```python
from build123d import *

# Parameters (mm, degrees)
ESQUISSE1_R        = 11.5
ESQUISSE1_R_2      = 1.6
BOSS_EXTRU_1_DEPTH = 4.8


with BuildPart() as part:
    # Esquisse1 → Boss.-Extru.1 (new body)
    with BuildSketch(Plane(origin=(0, 0, 0), x_dir=(-1, 0, 0), z_dir=(0, 0, -1))):
        with BuildLine():
            Line((0, 9.500081158), (0, 49.000418249))
            ThreePointArc((0, 49.000418249), (-1.464478579, 52.535982296), (-5.000042626, 54.000460875))
            Line((-5.000042626, 54.000460875), (-68.000581364, 54.000460875))
            ThreePointArc((-68.000581364, 54.000460875), (-71.53614516, 52.535982401), (-73.000623635, 49.000418605))
            Line((-73.000623635, 49.000418605), (-73.000623635, 9.500081158))
            ThreePointArc((-73.000623635, 9.500081158), (-72.854175775, 9.146524747), (-72.500619364, 9.000076887))
            Line((-72.500619364, 9.000076887), (-47.250403654, 9.000076887))
            Line((-47.250403654, 9.000076887), (-47.250403654, 1.000007743))
            ThreePointArc((-47.250403654, 1.000007743), (-46.95750587, 0.292889941), (-46.250388068, -7.843e-06))
            Line((-46.250388068, -7.843e-06), (-26.75023547, -7.843e-06))
            ThreePointArc((-26.75023547, -7.843e-06), (-26.043121781, 0.292888237), (-25.750225701, 1.000001925))
            Line((-25.750225701, 1.000001925), (-25.750225701, 9.000076887))
            Line((-25.750225701, 9.000076887), (-0.500004271, 9.000076887))
            ThreePointArc((-0.500004271, 9.000076887), (-0.14644786, 9.146524747), (0, 9.500081158))
        make_face()
        with Locations((-36.5004012, 30.150219609)):
            Circle(ESQUISSE1_R, mode=Mode.SUBTRACT)
        with Locations((-52.0004012, 14.650219609)):
            Circle(ESQUISSE1_R_2, mode=Mode.SUBTRACT)
        with Locations((-52.000444233, 45.650219609)):
            Circle(ESQUISSE1_R_2, mode=Mode.SUBTRACT)
        with Locations((-21.0004012, 14.650219609)):
            Circle(ESQUISSE1_R_2, mode=Mode.SUBTRACT)
        with Locations((-21.0004012, 45.650219609)):
            Circle(ESQUISSE1_R_2, mode=Mode.SUBTRACT)
        Polygon((-6.200052966, 47.036041823), (-5.614406963, 46.45039682), (-5.400046132, 45.650389986), (-5.614406963, 44.850383151), (-6.200052966, 44.264738148), (-7.000059801, 44.050376317), (-7.800066635, 44.264738148), (-8.385711638, 44.850383151), (-8.600073469, 45.650389986), (-8.385711638, 46.45039682), (-7.800066635, 47.036041823), (-7.000059801, 47.250403654), align=None, mode=Mode.SUBTRACT)
        Polygon((-4.750040579, 35.000299003), (-4.716546293, 35.125300071), (-4.625039511, 35.216810853), (-4.500038443, 35.250301139), (-4.375037375, 35.216810853), (-4.283530594, 35.125300071), (-4.250036308, 35.000299003), (-4.283530594, 34.875297935), (-4.375037375, 34.783787154), (-4.500038443, 34.750296868), (-4.500038443, 25.250215709), (-4.375037375, 25.216725423), (-4.283530594, 25.125214642), (-4.250036308, 25.000213574), (-4.283530594, 24.875212506), (-4.375037375, 24.783701724), (-4.500038443, 24.750211438), (-4.625039511, 24.783701724), (-4.716546293, 24.875212506), (-4.750040579, 25.000213574), (-9.250079022, 25.000213574), (-9.283572308, 24.875212506), (-9.37508009, 24.783701724), (-9.500081158, 24.750211438), (-9.625082226, 24.783701724), (-9.716589008, 24.875212506), (-9.750083294, 25.000213574), (-9.716589008, 25.125214642), (-9.625082226, 25.216725423), (-9.500081158, 25.250215709), (-9.500081158, 34.750296868), (-9.625082226, 34.783787154), (-9.716589008, 34.875297935), (-9.750083294, 35.000299003), (-9.716589008, 35.125300071), (-9.625082226, 35.216810853), (-9.500081158, 35.250301139), (-9.37508009, 35.216810853), (-9.283572308, 35.125300071), (-9.250079022, 35.000299003), align=None, mode=Mode.SUBTRACT)
        Polygon((-5.614406963, 15.450131989), (-5.400046132, 14.650125154), (-5.614406963, 13.85011832), (-6.200052966, 13.264473317), (-7.000059801, 13.050111485), (-7.800066635, 13.264473317), (-8.385711638, 13.85011832), (-8.600073469, 14.650125154), (-8.385711638, 15.450131989), (-7.800066635, 16.035776992), (-7.000059801, 16.250138823), (-6.200052966, 16.035776992), align=None, mode=Mode.SUBTRACT)
        Polygon((-30.100257143, 1.874182011), (-30.750262696, 1.700013523), (-31.400268249, 1.874182011), (-31.876102314, 2.350020076), (-32.050273802, 3.000025629), (-31.876102314, 3.650030182), (-31.400268249, 4.125868247), (-30.750262696, 4.300036735), (-30.100257143, 4.125868247), (-29.624423078, 3.650030182), (-29.45025159, 3.000025629), (-29.624423078, 2.350020076), align=None, mode=Mode.SUBTRACT)
        Polygon((-39.600338301, 1.874182011), (-40.250343854, 1.700013523), (-40.900349407, 1.874182011), (-41.376193472, 2.350020076), (-41.55035496, 3.000025629), (-41.376193472, 3.650030182), (-40.900349407, 4.125868247), (-40.250343854, 4.300036735), (-39.600338301, 4.125868247), (-39.124504236, 3.650030182), (-38.950332748, 3.000025629), (-39.124504236, 2.350020076), align=None, mode=Mode.SUBTRACT)
        Polygon((-64.400550166, 14.650125154), (-64.614911997, 13.85011832), (-65.200557, 13.264473317), (-66.000563835, 13.050111485), (-66.800570669, 13.264473317), (-67.386215672, 13.85011832), (-67.600577503, 14.650125154), (-67.386215672, 15.450131989), (-66.800570669, 16.035776992), (-66.000563835, 16.250138823), (-65.200557, 16.035776992), (-64.614911997, 15.450131989), align=None, mode=Mode.SUBTRACT)
        Polygon((-63.625543545, 24.783701724), (-63.717054327, 24.875212506), (-63.750544613, 25.000213574), (-68.250583056, 25.000213574), (-68.284073342, 24.875212506), (-68.375584124, 24.783701724), (-68.500585192, 24.750211438), (-68.62558626, 24.783701724), (-68.717097042, 24.875212506), (-68.750587328, 25.000213574), (-68.717097042, 25.125214642), (-68.62558626, 25.216725423), (-68.500585192, 25.250215709), (-68.500585192, 34.750296868), (-68.62558626, 34.783787154), (-68.717097042, 34.875297935), (-68.750587328, 35.000299003), (-68.717097042, 35.125300071), (-68.62558626, 35.216810853), (-68.500585192, 35.250301139), (-68.375584124, 35.216810853), (-68.284073342, 35.125300071), (-68.250583056, 35.000299003), (-63.750544613, 35.000299003), (-63.717054327, 35.125300071), (-63.625543545, 35.216810853), (-63.500542477, 35.250301139), (-63.375541409, 35.216810853), (-63.284040628, 35.125300071), (-63.250540342, 35.000299003), (-63.284040628, 34.875297935), (-63.375541409, 34.783787154), (-63.500542477, 34.750296868), (-63.500542477, 25.250215709), (-63.375541409, 25.216725423), (-63.284040628, 25.125214642), (-63.250540342, 25.000213574), (-63.284040628, 24.875212506), (-63.375541409, 24.783701724), (-63.500542477, 24.750211438), align=None, mode=Mode.SUBTRACT)
        Polygon((-66.800570669, 47.036041823), (-66.000563835, 47.250403654), (-65.200557, 47.036041823), (-64.614911997, 46.45039682), (-64.400550166, 45.650389986), (-64.614911997, 44.850383151), (-65.200557, 44.264738148), (-66.000563835, 44.050376317), (-66.800570669, 44.264738148), (-67.386215672, 44.850383151), (-67.600577503, 45.650389986), (-67.386215672, 46.45039682), align=None, mode=Mode.SUBTRACT)
    extrude(amount=-BOSS_EXTRU_1_DEPTH)


solid = part.part
```
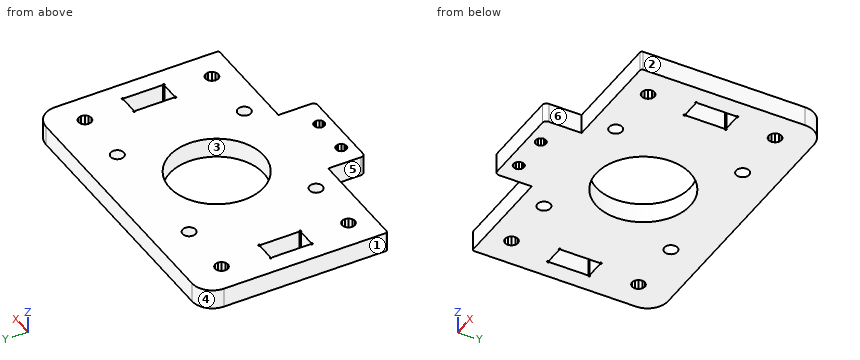
Source: CAD feature listing. Evaluate the final solid. Frame: model axes, mm. Face numbers are marked on the shaded views. A direction names the side the tool comes from. Give positions to 0.01 mm unless a question says otherwise; leave off trailing zeros. Write each loop counter-clockwise with the first axis right and the second up, starting at its lowest first coordinate (ties: lowest second). Pieces come first, ordered by that corner, then holes.
1. Section query D-D (x = 52.5). Return the cut outline in (y, z).
2. Section query A-A (x = 37). Return the cut outline in (y, z).
3. Section query C-C (y = 34). Return the cut outline in (x, z).
4. Section query B-B (y = 20). Return the cut outline in (x, z), then the cut area to 3 significant figures.
5. Material intervals for line 1 along X through (y, z) = (15.5, 3.45); line 2 along Y through (x, z) = (37, 0.4); line 3 along X through (y, z) = (33, 0.45), sorted ascending.
6. Pull-direction query (X, two-part tool) for the marked faces 1, 2 and 3; classes: +X half, -X half, draft (parallel to the pull), parting line (faces both ways), or undercut.
7. First-contact query: pin 1 (1.5 mm diameter, centred on x = 62.5, z = 2, fed in from -Y). Flat tip, straight axial feed; report the tip coordinate or a pass-through.
8. Access query for the marked faces 4, 5 and 6. Directions: +Z, -Z, +X, -X, +Y, -Y. A direction counts if a zero-diameter tool reaches every point of the face in a straight line with its end or side. Return the directions, or none.
Output values:
1. outline: (9, 0) - (13.13, 0) - (13.13, 4.8) - (9, 4.8) - close; (16.17, 0) - (44.13, 0) - (44.13, 4.8) - (16.17, 4.8) - close; (47.17, 0) - (54, 0) - (54, 4.8) - (47.17, 4.8) - close
2. outline: (0, 0) - (18.66, 0) - (18.66, 4.8) - (0, 4.8) - close; (41.64, 0) - (54, 0) - (54, 4.8) - (41.64, 4.8) - close
3. outline: (0, 0) - (4.5, 0) - (4.5, 4.8) - (0, 4.8) - close; (9.5, 0) - (25.66, 0) - (25.66, 4.8) - (9.5, 4.8) - close; (47.34, 0) - (63.5, 0) - (63.5, 4.8) - (47.34, 4.8) - close; (68.5, 0) - (73, 0) - (73, 4.8) - (68.5, 4.8) - close
4. outline: (0, 0) - (31.09, 0) - (31.09, 4.8) - (0, 4.8) - close; (41.91, 0) - (73, 0) - (73, 4.8) - (41.91, 4.8) - close
4. area: 299 mm2
5. line 1: x = 0 to 5.66, 8.34 to 19.64, 22.36 to 50.64, 53.36 to 64.66, 67.34 to 73
5. line 2: y = 0 to 18.66, 41.64 to 54
5. line 3: x = 0 to 4.5, 9.5 to 25.36, 47.64 to 63.5, 68.5 to 73
6. face 1: -X half
6. face 2: +X half
6. face 3: undercut
7. pin 1: stops at y = 9
8. face 4: +Z, -Z, -X, +Y
8. face 5: +Z, -Z, -X, -Y
8. face 6: +Z, -Z, +X, -Y
